Could you check a few things on this model? Use its own coordinates, in mm. A direction names the side the tool comes from. Give positions to 0.01 mm unless a question says otherwise; leave off trailing zeros. Order: outer loops, then holes, each group sorted by start corner. A loop starts at its lowest first (then second) coordinate and runs counter-clockwise, first axis right, second up.
from build123d import *

# Parameters (mm, degrees)
SKETCH1_R           = 1.3
BOSS_EXTRUDE1_DEPTH = 9
CUT_REVOLVE3_ANGLE  = 180
SKETCH8_R           = 7.6
CUT_EXTRUDE4_DEPTH  = 5.5
SKETCH9_R           = 2.65
CUT_EXTRUDE5_DEPTH  = 52.660312042
BOSS_EXTRUDE7_DEPTH = 9
CUT_REVOLVE4_ANGLE  = 180
FILLET1_R           = 6
FILLET2_R           = 4
FILLET3_R           = 3
FILLET4_R           = 3


with BuildPart() as part:
    # Sketch1 → Boss-Extrude1 (new body)
    with BuildSketch(Plane(origin=(0, 0, 0), x_dir=(0, 0, -1), z_dir=(1, 0, 0))):
        Polygon((0, -20), (22.5, -24.769696007), (45, -20), (45, 0), (22.5, 4.769696007), (0, 0), align=None)
        with Locations((22.5, -20.680807118)):
            Circle(SKETCH1_R, mode=Mode.SUBTRACT)
        with Locations((22.5, 0.680807118)):
            Circle(SKETCH1_R, mode=Mode.SUBTRACT)
        with Locations((42, -17)):
            Circle(SKETCH1_R, mode=Mode.SUBTRACT)
        with Locations((3, -17)):
            Circle(SKETCH1_R, mode=Mode.SUBTRACT)
        with Locations((3, -3)):
            Circle(SKETCH1_R, mode=Mode.SUBTRACT)
        with Locations((42, -3)):
            Circle(SKETCH1_R, mode=Mode.SUBTRACT)
    extrude(amount=BOSS_EXTRUDE1_DEPTH)

    # Sketch7 → Cut-Revolve3 (revolve, cut)
    with BuildSketch(Plane.ZY):
        with BuildLine():
            Line((-41.7, -10), (-31.3, -10))
            ThreePointArc((-31.3, -10), (-36.5, -4.8), (-41.7, -10))
        make_face()
        with BuildLine():
            Line((-13.7, -10), (-3.3, -10))
            ThreePointArc((-3.3, -10), (-8.5, -4.8), (-13.7, -10))
        make_face()
    revolve(axis=Axis((0, -10, -41.7), (0, 0, -1)), revolution_arc=CUT_REVOLVE3_ANGLE, mode=Mode.SUBTRACT)

    # Sketch8 → Cut-Extrude4 (cut)
    with BuildSketch(Plane.ZY):
        with Locations((-22.5, -10)):
            Circle(SKETCH8_R)
    extrude(amount=-CUT_EXTRUDE4_DEPTH, mode=Mode.SUBTRACT)

    # Sketch9 → Cut-Extrude5 (cut, through all)
    with BuildSketch(Plane.ZY.offset(-5.5)):
        with Locations((-22.5, -10)):
            Circle(SKETCH9_R)
    extrude(amount=-CUT_EXTRUDE5_DEPTH, mode=Mode.SUBTRACT)

    # Sketch16 → Boss-Extrude7 (add)
    with BuildSketch(Plane(origin=(9, 0, 0), x_dir=(0, 0, -1), z_dir=(1, 0, 0))):
        Polygon((38.152173913, -21.451646611), (38.152173913, -38.451646611), (23.152173913, -38.451646611), (23.152173913, -24.631443949), align=None)
    extrude(amount=-BOSS_EXTRUDE7_DEPTH)

    # Sketch17 → Cut-Revolve4 (revolve, cut)
    with BuildSketch(Plane.ZY):
        with BuildLine():
            Line((-25.452173913, -30.451646611), (-35.852173913, -30.451646611))
            ThreePointArc((-35.852173913, -30.451646611), (-30.652173913, -25.251646611), (-25.452173913, -30.451646611))
        make_face()
    revolve(axis=Axis((0, -30.451646611, -25.452173913), (0, 0, -1)), revolution_arc=CUT_REVOLVE4_ANGLE, mode=Mode.SUBTRACT)

    # Fillet1
    fillet1_edges = [part.edges().sort_by_distance(p)[0] for p in [
        (4.5, -38.451646611, -38.152173913),
        (4.5, -38.451646611, -23.152173913),
    ]]
    fillet(fillet1_edges, radius=FILLET1_R)

    # Fillet2
    fillet2_edges = [part.edges().sort_by_distance(p)[0] for p in [
        (4.5, -20, -45),
        (4.5, -20, 0),
        (4.5, 0, 0),
        (4.5, 0, -45),
    ]]
    fillet(fillet2_edges, radius=FILLET2_R)

    # Fillet3
    # the kernel refuses this fillet: 3 mm, written as the material it adds along each edge
    with BuildSketch(Plane(origin=(9, -24.631443949, -23.152173913), x_dir=(0, -0.20737808726534282, 0.9782608695650501), z_dir=(-1, 0, 0))) as fillet3_piece_1:
        with BuildLine():
            CenterArc((3.350740319, -1.340055458), FILLET3_R, 153.468795145, 38.499950409)
            Line((0.41595771, -1.96218972), (0.357262058, -1.974632405))
            Line((0.357262058, -1.974632405), (-0.058695652, -0.012442685))
            Line((-0.058695652, -0.012442685), (0, 0.06))
            ThreePointArc((0, 0.06), (0.333333333, 0.06), (0.612985194, 0.026801109))
            Line((0.612985194, 0.026801109), (0.666666667, 0))
        make_face()
    extrude(amount=9)
    with BuildSketch(Plane(origin=(9, -21.451646611, -38.152173913), x_dir=(0, -1, 0), z_dir=(-1, 0, 0))) as fillet3_piece_2:
        with BuildLine():
            CenterArc((FILLET3_R * 0.810235733018, -FILLET3_R), FILLET3_R, 90, 78.031254445)
            Line((-FILLET3_R * 0.168025136547, -FILLET3_R * 0.792621912735), (-FILLET3_R * 0.187590353938, -FILLET3_R * 0.78847435099))
            Line((-FILLET3_R * 0.187590353938, -FILLET3_R * 0.78847435099), (-FILLET3_R * 0.0162047146604, FILLET3_R * 0.02))
            Line((-FILLET3_R * 0.0162047146604, FILLET3_R * 0.02), (FILLET3_R * 0.810235733018, FILLET3_R * 0.02))
            Line((FILLET3_R * 0.810235733018, FILLET3_R * 0.02), (FILLET3_R * 0.810235733018, 0))
        make_face()
    extrude(amount=9)

    # Fillet4
    fillet4_edges = [part.edges().sort_by_distance(p)[0] for p in [
        (4.5, -24.769696007, -22.5),
    ]]
    fillet(fillet4_edges, radius=FILLET4_R)


solid = part.part
Item 1: Imagine slicing it at A-A on y = -10. List the corners of the cut face in (x, z) for me, then the cut area to 3 significant figures.
Findings:
outline: (0, -45) - (9, -45) - (9, -25.15) - (5.5, -25.15) - (5.5, -30.1) - (0, -30.1) - (0, -31.3) arc R5.2 cw to (0, -41.7) - close; (0, -14.9) - (5.5, -14.9) - (5.5, -19.85) - (9, -19.85) - (9, 0) - (0, 0) - (0, -3.3) arc R5.2 cw to (0, -13.7) - close
area: 218 mm2
Item 2: For faces 4 (the cylindrical face through (4.44, -16.94, -40.7)), 5 (the cylindrical face through (2.712, -9.666, -30.093)), which set-ups out of +Z, -Z, +X, -X, +Y, -Y let a thin tool reach every point of the face, with its end or its side?
Findings:
face 4: +X, -X
face 5: -X
Item 3: For pin 1 (9 mm diameter, centred on y = -10, z = -22.5, fed in from -X); pin 2 (2 mm diameter, centred on x = 1.5, y = -2, fed in from -Z); pin 3 (5 mm diameter, centred on x = 2, z = -10.5, fed in from +Y), each with a flat end and sliding along its axis, tell me the tip position at first contact or that it passes through.
Findings:
pin 1: stops at x = 5.5
pin 2: stops at z = -44.99
pin 3: stops at y = 2.76
Item 4: Imagine slicing it at D-D on y = -31. List the corners of the cut face in (x, z) for me.
Findings:
outline: (0, -38.15) - (9, -38.15) - (9, -23.15) - (0, -23.15) - (0, -25.48) arc R5.17 cw to (0, -35.82) - close
Item 5: Imagine slicing it at C-C on x = 1.5. Give the number of separate pieces and of enclosed holes in the cut face, then the cut area to 3 significant figures.
Findings:
separate pieces: 1
enclosed holes: 10
area: 878 mm2
Item 6: Imagine slicing it at B-B on z = -16. List the corners of the cut face in (x, y) for me.
Findings:
outline: (0, -23.39) - (9, -23.39) - (9, 3.39) - (0, 3.39) - (0, -6.06) - (5.5, -6.06) - (5.5, -13.94) - (0, -13.94) - close
Item 7: We'd pull the mould along Z, two halves only. Please class faces 1 (the flat face through (5, -30, -23.152)), 2 (the cylindrical face through (4.56, -19.31, -44.08)), 3 (the cylindrical face through (4.4, 0.7, -21.2)): +Z half, -Z half, draft (parallel to the pull), parting line (faces both ways), or undercut.
Findings:
face 1: +Z half
face 2: -Z half
face 3: undercut
Item 8: Please list where these lines run through material, in increasing order: line 1 along Z through (x, y) = (6.75, -2.5); line 2 along Y through (x, z) = (4.5, -42); line 3 along Y through (x, z) = (3, -22.5).
Findings:
line 1: z = -44.93 to -43.2, -40.8 to -4.2, -1.8 to -0.07
line 2: y = -20.63 to -18.3, -15.7 to -4.3, -1.7 to 0.63
line 3: y = -25.47 to -21.98, -19.38 to -17.6, -2.4 to -0.62, 1.98 to 4.77
